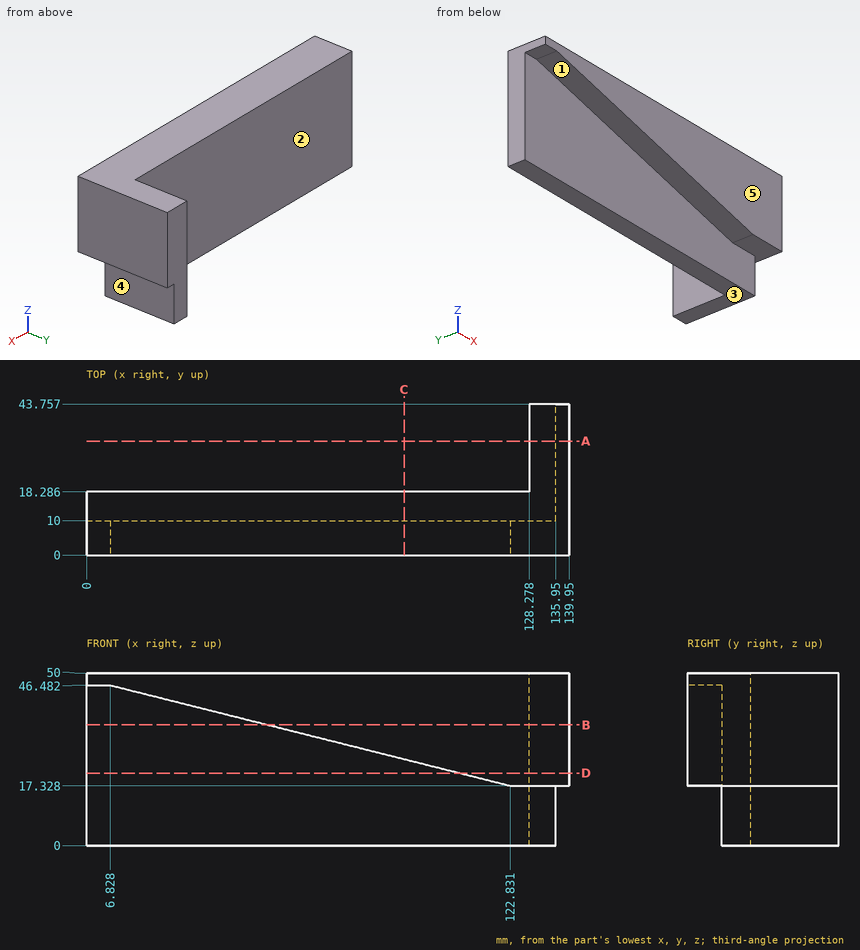
Could you check a few things on this drawing? It's one solid part, dimensions in mm from its lowest x, y, z. A direction names the side the tool comes from. Coordinates: 2 decimals unless noted, no trailing zeros. Order: outer loops, then holes, each group sorted by start corner. A loop starts at its lowest first (then second) coordinate and runs counter-clockwise, first axis right, second up. Notation, with made-up numbers: (80.25, -18) - (135.25, -18) arc R21 ccw to (135.25, -1) - close; hole circle Ø8 at (-13, 86). An arc over 180 degrees is marked (long way). Answer as a JSON object with one key per item and string values. Group by question number.
Q1. Imagine slicing it at A-A (y = 33). Please give me the cut outline in (x, z), and give its area (3 significant figures).
Q2. I need wall thicknesses on line 1 (X direction, y = 21, z = 35); line 2 (Y direction, x = 112.5, z = 22.5); line 3 (Y direction, x = 16.5, z = 25). Which ranges of each line are inside material? Lowest first, please. Write a range as from..to.
Q3. Imagine slicing it at B-B (z = 35). Please give me the cut outline in (x, y), and give its area (3 significant figures).
Q4. On a 3-axis mill with a long thin cutter (end or side, diameter ignored), from which of +Z, -Z, +X, -X, +Y, -Y can I reach the whole of each face in a straight line? I mean the marked faces 1, 2, 3, 4 and 5. Say none if no direction works.
Q5. Will these pins go through, and if not, where does the flat tip stop? P1, Ø7.5, axis at y = 31.5, z = 35, coming from the -X side; P2, Ø5.5, axis at x = 5, y = 3.5, coming from the -Z side; P3, Ø12, axis at x = 78.5, z = 26.5, coming from the +Y side.
Q6. Imagine slicing it at C-C (x = 92). Please give me the cut outline in (y, z).
Q7. Imagine slicing it at D-D (z = 21). Please give me the cut outline in (x, y).
Determined:
{
 "1": {"outline": "(128.28, 0) - (135.95, 0) - (135.95, 17.33) - (139.95, 17.33) - (139.95, 50) - (128.28, 50) - close", "area": "514 mm2"},
 "2": {"line 1": "x = 128.28..139.95", "line 2": "y = 0..18.29", "line 3": "y = 10..18.29"},
 "3": {"outline": "(0, 10) - (52.51, 10) - (52.51, 0) - (139.95, 0) - (139.95, 43.76) - (128.28, 43.76) - (128.28, 18.29) - (0, 18.29) - close", "area": "2,330 mm2"},
 "4": {"face 1": "-Z, -X, -Y", "face 2": "+Z, -Z, -X, +Y", "face 3": "-Z, +X, -X, +Y, -Y", "face 4": "-Z, +X, +Y, -Y", "face 5": "+Z, -Z, +X, -X, -Y"},
 "5": {"P1": "stops at x = 128.28", "P2": "stops at z = 46.25", "P3": "stops at y = 18.29"},
 "6": {"outline": "(0, 25.08) - (10, 25.08) - (10, 0) - (18.29, 0) - (18.29, 50) - (0, 50) - close"},
 "7": {"outline": "(0, 10) - (108.22, 10) - (108.22, 0) - (139.95, 0) - (139.95, 43.76) - (128.28, 43.76) - (128.28, 18.29) - (0, 18.29) - close"}
}
